Check sheet for the modelled part. Datum: model origin and axes. Units: mm. Face numbers are marked on the shaded views. A direction names the side the tool comes from. Round coordinates to 2 decimals unless told otherwise and drop trailing zeros. Write each loop counter-clockwise with the first axis right and the second up, starting at its lowest first coordinate (ties: lowest second). Pieces come first, ordered by that corner, then holes. Notation, with made-up numbers: (42.5, -25.75) - (97.5, -25.75) arc R23 ccw to (97.5, 11.25) - close; hole circle Ø7 at (-33, 29). An arc over 180 degrees is marked (long way). Use one line per item in the form item = value. Start each with the question number.
1) Section check A-A (x = 34). Record the boundary of the cut face in (y, z), then the cut area to 3 significant figures.
2) Gauge pin test, flat end, axial feed: P1, Ø4.5, axis at x = 34, y = 0, coming from the -Z side. Record the tip position at first contact, or that the pin passes through.
3) Set-up check for the marked faces 1 and 2: record each of +Z, -Z, +X, -X, +Y, -Y from which the full face is reachable in a straight line by a thin tool's end or side.
4) Section check B-B (x = -3). Record the boundary of the cut face in (y, z).
5) Scan lines: probe 1 along X at (y, z) = (3, -2); probe 2 along Y at (x, z) = (34, -0.5); probe 3 along Y at (x, z) = (34, -1). Record each from-to range of solid material in increasing order.
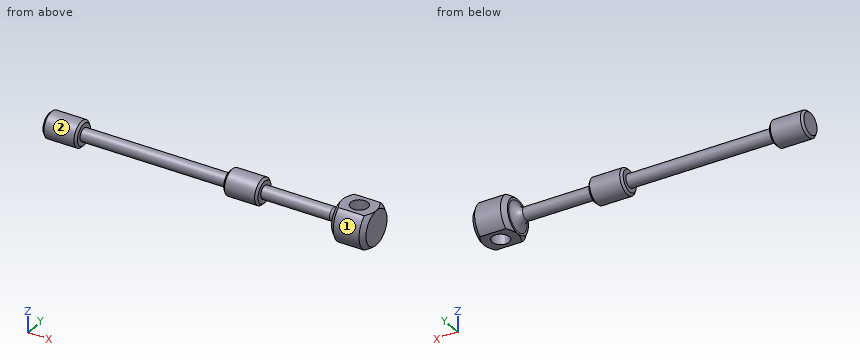
Solid Edge part; units mm, degrees
sketch "Sketch1" plane through (0, 0, 0) normal (1, 0, 0) x (0, 1, 0)
  circle A0 centre (0, 0) radius 1.5
extrude "Protrusion1" add sketch "Sketch1" along normal mid plane 76
sketch "Sketch2" plane through (-38, 0, 0) normal (-1, 0, 0) x (0, -1, 0)
  circle A0 centre (0, 0) radius 3
extrude "ExtrudedProtrusion_2" add sketch "Sketch2" against normal blind 8
sketch "Sketch3" plane through (8, 0, 0) normal (1, 0, 0) x (0, 1, 0)
  circle A0 centre (0, 0) radius 3
extrude "ExtrudedProtrusion_3" add sketch "Sketch3" along normal mid plane 8
chamfer "Chamfer_1" distance 0.5 angle 45 4 edges at (-38, 3, 0) (-30, 3, 0) (12, -3, 0) (4, -3, 0)
sketch "Sketch4" plane through (38, 0, 0) normal (1, 0, 0) x (0, 0, -1)
  circle A0 centre (0, 0) radius 5
extrude "ExtrudedProtrusion_4" add sketch "Sketch4" against normal blind 8
sketch "Sketch5" plane through (38, 0, 0) normal (1, 0, 0) x (0, 0, -1)
  line L0 (-4, -3) -> (-4, 3)
  arc A0 (-4, -3) -> (-4, 3) centre (0, 0) cw
  line L1 (4, -3) -> (4, 3)
  arc A1 (4, 3) -> (4, -3) centre (0, 0) cw
extrude "ExtrudedCutout_1" cut sketch "Sketch5" against normal blind 9
sketch "Sketch6" plane through (34, 0, 4) normal (0, 0, 1) x (1, 0, 0)
  circle A0 centre (0, 0) radius 2
extrude "ExtrudedCutout_2" cut sketch "Sketch6" along normal mid plane 64.4682
chamfer "Chamfer_2" distance 1 angle 45 2 edges at (30, -5, 0) (38, -5, 0)
chamfer "Chamfer_3" distance 1 angle 45 2 edges at (30, 5, 0) (38, 5, 0)
fillet "Round_1" radius 2 1 edges at (30, 1.5, 0)
Results are:
q1.outline = (-3, -4) - (-2, -4) - (-2, 4) - (-3, 4) arc R5 ccw to start; (2, -4) - (3, -4) arc R5 ccw to (3, 4) - (2, 4) - close
q1.area = 38.4 mm²
q2.P1 = -4
q3.face_1 = +X, -X, -Y
q3.face_2 = -X
q4.outline = circle Ø3 at (0, 0)
q5.probe_1 = 30 to 38
q5.probe_2 = -4.97 to -2, 2 to 4.97
q5.probe_3 = -4.9 to -2, 2 to 4.9
